Design review of the part built by this model. Coordinates are the model's own, in mm. Face numbers are marked on the shaded views. Give positions to 0.01 mm unless a question says otherwise; leave off trailing zeros. Write each loop counter-clockwise with the first axis right and the second up, starting at its lowest first coordinate (ties: lowest second). Pieces come first, ordered by that corner, then holes.
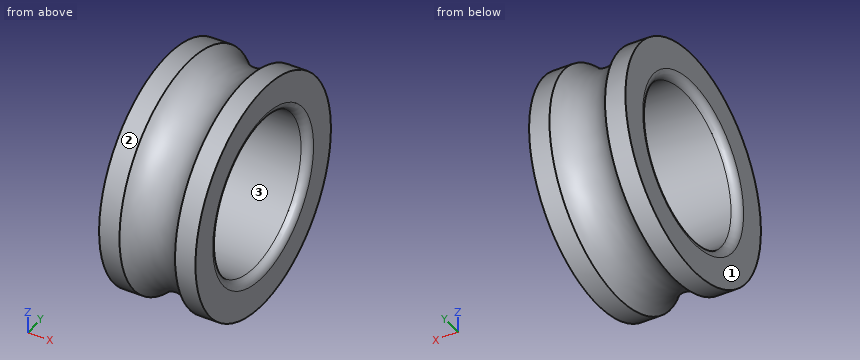
```python
from build123d import *

# Parameters (mm, degrees)
SCALE1_SCALE = 0.35


with BuildPart() as part:
    # Sketch1 → Revolve1 (revolve)
    with BuildSketch(Plane.XY, mode=Mode.PRIVATE) as revolve1_sk:
        with BuildLine():
            Line((-15.5, 37), (-8.94427191, 37))
            ThreePointArc((-8.94427191, 37), (0, 33), (8.94427191, 37))
            Line((8.94427191, 37), (15.5, 37))
            Line((15.5, 37), (15.5, 27.54))
            ThreePointArc((15.5, 27.54), (14.756051224, 25.743948776), (12.96, 25))
            Line((12.96, 25), (-12.96, 25))
            ThreePointArc((-12.96, 25), (-14.756051224, 25.743948776), (-15.5, 27.54))
            Line((-15.5, 27.54), (-15.5, 37))
        make_face()
    revolve(revolve1_sk.sketch.rotate(Axis((-21.666666667, 0, 0), (1, 0, 0)), 90), axis=Axis((-21.666666667, 0, 0), (1, 0, 0)))


with BuildPart() as part_1:
    # Scale1: scaled about (0, 0, 0)
    add(part.part.scale(SCALE1_SCALE))


solid = part_1.part
```
(1) To check wall thickness, follow L1, parallel to Y at x = 1.75, z = 0; L2, parallel to Z at x = -0.25, y = -2; L3, parallel to Y at x = 1, z = 0. State the ranges of each line that lie inside material, in increasing order.
Resolved:
L1: y = -11.93 to -8.75, 8.75 to 11.93
L2: z = -11.38 to -8.52, 8.52 to 11.38
L3: y = -11.67 to -8.75, 8.75 to 11.67
(2) Consider section C-C, the plane x = -4. Give the boundary of the cut face in (y, z).
Resolved:
outline: circle Ø25.9 at (0, 0); hole circle Ø17.5 at (0, 0)
(3) Clearance check with flat-ended pins moving along their axes: P1, Ø1.5, axis at x = 3, z = -3.5, coming from the +Y side; P2, Ø10, axis at y = -1, z = -7.5, coming from the -X side (3 decimals); P3, Ø5, axis at x = 3.5, z = -8.5, coming from the -Y side; P4, Ø6, axis at x = -0.5, y = -8.5, coming from the -Z side. State where each tip first meets the part, or that it passes through.
Resolved:
P1: stops at y = 12.65
P2: stops at x = -5.425
P3: stops at y = -11.48
P4: stops at z = -10.86
(4) Consider section D-D, the plane x = -2.25. Give the boundary of the cut face in (y, z).
Resolved:
outline: circle Ø24.41 at (0, 0); hole circle Ø17.5 at (0, 0)
(5) Mouldability with a two-part tool opening along Y and no side actions: class the marked faces 1, 2 and 3 as pulls with the +Y half, pulls with the -Y half, needs draft (parallel to the pull), parting line crosses it, or undercut.
Resolved:
face 1: needs draft
face 2: parting line crosses it
face 3: undercut
